```python
from build123d import *

# Parameters (mm, degrees)
BOSS_EXTRUDE1_DEPTH = 7
CUT_EXTRUDE1_REACH  = 20.412
SKETCH3_R           = 1.55
CUT_EXTRUDE2_REACH  = 20.412
SKETCH4_R           = 1.55


with BuildPart() as part:
    # Sketch1 → Boss-Extrude1 (new body)
    with BuildSketch(Plane(origin=(0, 0, 0), x_dir=(1, 0, 0), z_dir=(0, 1, 0))):
        with BuildLine():
            Line((0, 0), (-13, 0))
            Line((-13, 0), (-13, 2))
            Line((-13, 2), (-6.242640687, 2))
            ThreePointArc((-6.242640687, 2), (-5.09459039, 2.228361402), (-4.121320344, 2.878679656))
            Line((-4.121320344, 2.878679656), (-2.878679656, 4.121320344))
            ThreePointArc((-2.878679656, 4.121320344), (-2.228361402, 5.09459039), (-2, 6.242640687))
            Line((-2, 6.242640687), (-2, 13))
            Line((-2, 13), (0, 13))
            Line((0, 13), (0, 0))
        make_face()
    extrude(amount=BOSS_EXTRUDE1_DEPTH)

    # Sketch3 → Cut-Extrude1 (cut, up to next)
    with BuildSketch(Plane(origin=(0, 0, -2), x_dir=(-1, 0, 0), z_dir=(0, 0, -1)), mode=Mode.PRIVATE) as cut_extrude1_sk1:
        with Locations((9.621320344, 3.5)):
            Circle(SKETCH3_R)
    cut_extrude1_tool1 = extrude(cut_extrude1_sk1.sketch, amount=-CUT_EXTRUDE1_REACH, mode=Mode.PRIVATE) & part.part
    add(cut_extrude1_tool1.solids().sort_by_distance((-9.62132, 3.5, -2))[0], mode=Mode.SUBTRACT)

    # Sketch4 → Cut-Extrude2 (cut, up to next)
    with BuildSketch(Plane.ZY.offset(2), mode=Mode.PRIVATE) as cut_extrude2_sk1:
        with Locations((-9.621320344, 3.5)):
            Circle(SKETCH4_R)
    cut_extrude2_tool1 = extrude(cut_extrude2_sk1.sketch, amount=-CUT_EXTRUDE2_REACH, mode=Mode.PRIVATE) & part.part
    add(cut_extrude2_tool1.solids().sort_by_distance((-2, 3.5, -9.62132))[0], mode=Mode.SUBTRACT)


solid = part.part
```
Read the model definition and answer for the solid it produces. Units are mm, in the model's axes. A direction names the side the tool comes from. Coordinates: 2 decimals unless noted, no trailing zeros. Write each loop counter-clockwise with the first axis right and the second up, starting at its lowest first coordinate (ties: lowest second). Pieces come first, ordered by that corner, then holes. Notation, with made-up numbers: (70.5, 52) -> (109.5, 52) arc R14 ccw to (109.5, 59) -> close; hole circle Ø1 at (61, 12.5). An arc over 180 degrees is marked (long way). Return JSON: item names as keys, results as strings.
1. Determine the mould class of faces 1 (the face through (0, 3, -7)), 2 (the face through (-1.014, 2.557, -10.851)), 3 (the face through (-6, 3, 0)) for opening direction Z: pulls with the +Z half, pulls with the -Z half, needs draft (parallel to the pull), parting line crosses it, or undercut.
Found:
{"face 1": "needs draft", "face 2": "undercut", "face 3": "pulls with the +Z half"}
2. A cutting plane is placed at A-A (y = 3.5). Determine the outline of the cut face in (x, z).
Found:
{"outline": "(-13, -2) -> (-11.17, -2) -> (-11.17, 0) -> (-13, 0) -> close; (-8.07, -2) -> (-6.24, -2) arc R3 cw to (-4.12, -2.88) -> (-2.88, -4.12) arc R3 cw to (-2, -6.24) -> (-2, -8.07) -> (0, -8.07) -> (0, 0) -> (-8.07, 0) -> close; (-2, -13) -> (0, -13) -> (0, -11.17) -> (-2, -11.17) -> close"}
3. A cutting plane is placed at C-C (x = -8.75). Determine the outline of the cut face in (y, z).
Found:
{"outline": "(0, -2) -> (2.22, -2) -> (2.22, 0) -> (0, 0) -> close; (4.78, -2) -> (7, -2) -> (7, 0) -> (4.78, 0) -> close"}
4. A cutting plane is placed at D-D (y = 1). Determine the outline of the cut face in (x, z).
Found:
{"outline": "(-13, -2) -> (-6.24, -2) arc R3 cw to (-4.12, -2.88) -> (-2.88, -4.12) arc R3 cw to (-2, -6.24) -> (-2, -13) -> (0, -13) -> (0, 0) -> (-13, 0) -> close"}
5. Each of these flat-tipped pins is pushed along its axis until it touches: P1, Ø2.5, axis at y = 3.5, z = -9.62, coming from the +X side (1 decimal); P2, Ø3.5, axis at x = -8.5, y = 3, coming from the -Z side. Where does it stop, or does it pass through?
Found:
{"P1": "through", "P2": "z = -2"}
6. Find the intervals of material crossed by line 1 along Z through (x, y) = (-8, 5.5); line 2 along X through (y, z) = (4.5, -1.25), in increasing order. Write a range as from..to.
Found:
{"line 1": "-2..0", "line 2": "-13..-10.81, -8.44..0"}
7. A tool of negligible diameter and unlimited length cuts with its end or side. For faces 4 (the face through (-13, 3, -1)), 5 (the face through (-2, 2.7, -8.1)), from which of +Z, -Z, +X, -X, +Y, -Y can it reach the whole face along a straight path? Write none if from no direction.
Found:
{"face 4": "+Z, -Z, -X, +Y, -Y", "face 5": "-Z, -X, +Y, -Y"}
8. A cutting plane is placed at B-B (z = -1.25). Determine the outline of the cut face in (x, y), and give its area (3 significant figures).
Found:
{"outline": "(-13, 0) -> (0, 0) -> (0, 7) -> (-13, 7) -> close; hole circle Ø3.1 at (-9.62, 3.5)", "area": "83.5 mm2"}
